Read the model definition and answer for the solid it produces. Units are mm, in the model's axes. Give positions to 0.01 mm unless a question says otherwise; leave off trailing zeros. Order: outer loops, then holes, each group sorted by start corner. A loop starts at its lowest first (then second) coordinate and runs counter-clockwise, first axis right, second up. Notation, with made-up numbers: M 4,28.25 L 35,28.25 A7 ccw 35,36.25 Z; hole C 38,-10 d11. An arc over 180 degrees is marked long. One line per item, written item: value.
from build123d import *

# Parameters (mm, degrees)
F_01_START                                = 7.48
S01_INSTALLED_SPRING_CLIP_ENVELOPE_R      = 4.65
S01_INSTALLED_SPRING_CLIP_ENVELOPE_R_2    = 2.01
F_01_INSTALLED_SPRING_CLIP_ENVELOPE_DEPTH = 0.7
F_02_START                                = 7.46
S02_RADIAL_ENTRY_OPENING_W                = 3.34
S02_RADIAL_ENTRY_OPENING_H                = 5.1
F_02_RADIAL_ENTRY_OPENING_DEPTH           = 0.75
F_03_START                                = 7.46
S03_LEFT_SPRING_RELIEF_R                  = 1.06
F_03_LEFT_SPRING_RELIEF_DEPTH             = 0.75
F_04_START                                = 7.46
S04_RIGHT_SPRING_RELIEF_R                 = 1.06
F_04_RIGHT_SPRING_RELIEF_DEPTH            = 0.75


with BuildPart() as part:
    # S01 - Installed spring clip envelope → 01 - Installed spring clip envelope (new body)
    with BuildSketch(Plane.XY.offset(F_01_START)):
        Circle(S01_INSTALLED_SPRING_CLIP_ENVELOPE_R)
        Circle(S01_INSTALLED_SPRING_CLIP_ENVELOPE_R_2, mode=Mode.SUBTRACT)
    extrude(amount=F_01_INSTALLED_SPRING_CLIP_ENVELOPE_DEPTH)

    # S02 - Radial entry opening → 02 - Radial entry opening (cut)
    with BuildSketch(Plane.XY.offset(F_02_START)):
        with Locations((0, -2.25)):
            Rectangle(S02_RADIAL_ENTRY_OPENING_W, S02_RADIAL_ENTRY_OPENING_H)
    extrude(amount=F_02_RADIAL_ENTRY_OPENING_DEPTH, mode=Mode.SUBTRACT)

    # S03 - Left spring relief → 03 - Left spring relief (cut)
    with BuildSketch(Plane.XY.offset(F_03_START)):
        with Locations((-1.95, 0.95)):
            Circle(S03_LEFT_SPRING_RELIEF_R)
    extrude(amount=F_03_LEFT_SPRING_RELIEF_DEPTH, mode=Mode.SUBTRACT)

    # S04 - Right spring relief → 04 - Right spring relief (cut)
    with BuildSketch(Plane.XY.offset(F_04_START)):
        with Locations((1.95, 0.95)):
            Circle(S04_RIGHT_SPRING_RELIEF_R)
    extrude(amount=F_04_RIGHT_SPRING_RELIEF_DEPTH, mode=Mode.SUBTRACT)


solid = part.part
1) Find section C-C, the plane y = 0.75. Write down the section's boundary in (x, z), plus the area to 3 significant figures.
Reported:
outline: M -4.59,7.48 L -2.99,7.48 L -2.99,8.18 L -4.59,8.18 Z; M 2.99,7.48 L 4.59,7.48 L 4.59,8.18 L 2.99,8.18 Z
area: 2.24 mm^2
2) Consider probe 1 along X at (y, z) = (0.95, 8); probe 2 along X at (y, z) = (-2.25, 7.85); probe 3 along Y at (x, z) = (2.5, 8). Determine where each line is inside the solid, lowest interval first.
Reported:
probe 1: x = -4.55 to -3.01, 3.01 to 4.55
probe 2: x = -4.07 to -1.67, 1.67 to 4.07
probe 3: y = -3.92 to 0.04, 1.86 to 3.92
3) Determine the mould class of faces 1 (the face through (0.181, 4.646, 7.825)), 2 (the face through (-0.1, 2.2, 8.18)), 3 (the face through (-2.89, 1.44, 7.83)) for opening direction Y: +Y half, -Y half, draft (parallel to the pull), parting line (faces both ways), or undercut.
Reported:
face 1: parting line
face 2: draft
face 3: undercut
4) Find section A-A, the plane y = -3.5. Write down the section's boundary in (x, z).
Reported:
outline: M -3.06,7.48 L -1.67,7.48 L -1.67,8.18 L -3.06,8.18 Z; M 1.67,7.48 L 3.06,7.48 L 3.06,8.18 L 1.67,8.18 Z
5) This flat-tipped pin is pushed along its axis until it touches: pin 1 Ø1.7 at (x, y) = (1.95, 0.95) entering from -Z. Where does it stop, or does it pass through?
Reported:
pin 1: passes through
6) Find section D-D, the plane x = -3.5. Write down the section's boundary in (y, z).
Reported:
outline: M -3.06,7.48 L 3.06,7.48 L 3.06,8.18 L -3.06,8.18 Z
7) Find section B-B, the plane z = 7.7. Write down the section's boundary in (x, y), plus the area to 3 significant figures.
Reported:
outline: M -2.01,-0.11 A1.06 cw long -1.15,1.65 A2.01 cw 1.15,1.65 A1.06 cw long 2.01,-0.11 A2.01 cw 1.67,-1.12 L 1.67,-4.34 A4.65 ccw long -1.67,-4.34 L -1.67,-1.12 A2.01 cw Z
area: 41.3 mm^2
